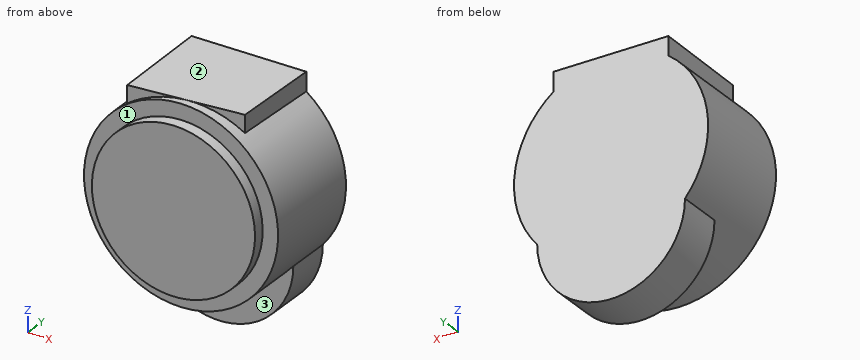
```python
from build123d import *

# Parameters (mm, degrees)
CROQUIS1_R              = 8.035
SALIENTE_EXTRUIR1_DEPTH = 1.15
CROQUIS2_R              = 9.56
SALIENTE_EXTRUIR2_DEPTH = 10.26
SALIENTE_EXTRUIR3_START = -4.46
SALIENTE_EXTRUIR3_DEPTH = 4.46
SALIENTE_EXTRUIR4_DEPTH = 4.46


with BuildPart() as part:
    # Croquis1 → Saliente-Extruir1 (new body)
    with BuildSketch(Plane(origin=(0, 0, 0), x_dir=(1, 0, 0), z_dir=(0, 1, 0))):
        with Locations(Location((0, 0, 0), (0, 0, 270))):
            Circle(CROQUIS1_R)
    extrude(amount=SALIENTE_EXTRUIR1_DEPTH)

    # Croquis2 → Saliente-Extruir2 (add)
    with BuildSketch(Plane(origin=(0, 1.15, 0), x_dir=(1, 0, 0), z_dir=(0, 1, 0))):
        with Locations(Location((0, 0, 0), (0, 0, 270))):
            Circle(CROQUIS2_R)
    extrude(amount=SALIENTE_EXTRUIR2_DEPTH)

    # Croquis3 → Saliente-Extruir3 (add)
    with BuildSketch(Plane(origin=(0, 11.41, 0), x_dir=(1, 0, 0), z_dir=(0, 1, 0)).offset(SALIENTE_EXTRUIR3_START)):
        with BuildLine():
            ThreePointArc((-7.280024761, 6.196356953), (0, 13.476381713), (7.280024761, 6.196356953))
            ThreePointArc((7.280024761, 6.196356953), (0, -9.56), (-7.280024761, 6.196356953))
        make_face()
    extrude(amount=SALIENTE_EXTRUIR3_DEPTH)

    # Croquis6 → Saliente-Extruir4 (add)
    with BuildSketch(Plane.XY.offset(9.56)):
        Polygon((-5.475, 1.41), (5.475, 2.41), (5.65, 11.41), (-5.65, 11.41), align=None)
    extrude(amount=-SALIENTE_EXTRUIR4_DEPTH)


solid = part.part
```
Verification items for the finished model (mm, model axes). Face numbers are marked on the shaded views. A direction names the side the tool comes from. Round coordinates to 2 decimals unless told otherwise and drop trailing zeros. Loops run counter-clockwise (first coordinate to the right, second up) from the corner with the lowest first, then second, coordinate; pieces in that order, holes last. Notation, with made-up numbers: (-39.5, -3) -> (14.5, -3) arc R19 ccw to (14.5, 11) -> close; hole circle Ø11 at (-28, 48.25). An arc over 180 degrees is marked (long way). Answer as a JSON object with one key per item and string values.
Q1. Go/stop test with flat-tipped pins: P1, Ø6, axis at x = -4.5, y = 2, coming from the -Z side; P2, Ø1.5, axis at x = -7, y = 7.5, coming from the +Z side. Record where each tip stops, or that it passes through.
Data:
{"P1": "stops at z = -9.44", "P2": "stops at z = 7.23"}
Q2. Section check A-A (z = 0). Record the boundary of the cut face in (x, y) (3 decimals).
Data:
{"outline": "(-9.56, 1.15) -> (-8.035, 1.15) -> (-8.035, 0) -> (8.035, 0) -> (8.035, 1.15) -> (9.56, 1.15) -> (9.56, 11.41) -> (-9.56, 11.41) -> close"}
Q3. Section check D-D (z = 5.5). Record the boundary of the cut face in (x, y).
Data:
{"outline": "(-7.82, 1.15) -> (-5.86, 1.15) -> (-5.86, 0) -> (5.86, 0) -> (5.86, 1.15) -> (7.82, 1.15) -> (7.82, 11.41) -> (-7.82, 11.41) -> close"}
Q4. Section check B-B (x = -4.25). Record the boundary of the cut face in (y, z).
Data:
{"outline": "(0, -6.82) -> (1.15, -6.82) -> (1.15, -8.56) -> (6.95, -8.56) -> (6.95, -12.11) -> (11.41, -12.11) -> (11.41, 9.56) -> (1.52, 9.56) -> (1.52, 8.56) -> (1.15, 8.56) -> (1.15, 6.82) -> (0, 6.82) -> close"}
Q5. Section check C-C (x = -2). Record the boundary of the cut face in (y, z), then the cut area to 3 significant figures.
Data:
{"outline": "(0, -7.78) -> (1.15, -7.78) -> (1.15, -9.35) -> (6.95, -9.35) -> (6.95, -13.2) -> (11.41, -13.2) -> (11.41, 9.56) -> (1.73, 9.56) -> (1.73, 9.35) -> (1.15, 9.35) -> (1.15, 7.78) -> (0, 7.78) -> close", "area": "229 mm2"}
Q6. Scan lines: line 1 (Y direction, x = -4.25, z = -8.25); line 2 (Z direction, x = -0.25, y = 10.5); line 3 (X direction, y = 9.5, z = -6.5). Record each from-to range of solid material in increasing order. Write a range as from..to.
Data:
{"line 1": "y = 1.15..11.41", "line 2": "z = -13.47..9.56", "line 3": "x = -7.27..7.27"}
Q7. Access from +Z, -Z, +X, -X, +Y, -Y to the whole of each face (thin tool, end or side, straight path). Record for the marked faces 1, 2 and 3.
Data:
{"face 1": "-Y", "face 2": "+Z, +X, -X, +Y, -Y", "face 3": "-Z, -Y"}
